from build123d import *

# Parameters (mm, degrees)
SKETCH1_W          = 16
SKETCH1_H          = 16
EXTRUDE1_DEPTH     = 8
SKETCH2_R          = 7.35
EXTRUDE2_DEPTH     = 7
SHELL1_T           = -1.3
SKETCH6_R          = 1
CUT_EXTRUDE1_DEPTH = 19.788294228
SKETCH4_R          = 1.15
EXTRUDE3_DEPTH     = 4
FILLET1_R          = 0.5
FILLET2_R          = 0.5
FILLET3_R          = 1


with BuildPart() as part:
    # Sketch1 → Extrude1 (new body)
    with BuildSketch(Plane.XY):
        Rectangle(SKETCH1_W, SKETCH1_H)
    extrude(amount=EXTRUDE1_DEPTH)

    # Sketch2 → Extrude2 (add)
    with BuildSketch(Plane.XY.offset(8)):
        Circle(SKETCH2_R)
    extrude(amount=EXTRUDE2_DEPTH)

    # Shell1
    shell1_openings = [part.faces().sort_by_distance(p)[0] for p in [
        (0, 0, 15),
        (0, 0, 0),
    ]]
    offset(amount=SHELL1_T, openings=shell1_openings, kind=Kind.INTERSECTION)

    # Sketch6 → Cut-Extrude1 (cut, through all)
    with BuildSketch(Plane(origin=(0, 0, 0), x_dir=(1, 0, 0), z_dir=(0, 1, 0))):
        with Locations(Location((0, -12.46, 0), (0, 0, 90))):
            Circle(SKETCH6_R)
    extrude(amount=CUT_EXTRUDE1_DEPTH, mode=Mode.SUBTRACT)

    # Sketch4 → Extrude3 (add)
    with BuildSketch(Plane.XY):
        with BuildLine():
            Line((-8, 1.9), (-10.3, 1.9))
            ThreePointArc((-10.3, 1.9), (-12.2, 0), (-10.3, -1.9))
            Line((-10.3, -1.9), (-8, -1.9))
            Line((-8, -1.9), (-8, 1.9))
        make_face()
        with Locations((-10.3, 0)):
            Circle(SKETCH4_R, mode=Mode.SUBTRACT)
        with BuildLine():
            Line((8, 1.9), (8, -1.9))
            Line((8, -1.9), (10.3, -1.9))
            ThreePointArc((10.3, -1.9), (12.2, 0), (10.3, 1.9))
            Line((10.3, 1.9), (8, 1.9))
        make_face()
        with Locations((10.3, 0)):
            Circle(SKETCH4_R, mode=Mode.SUBTRACT)
    extrude(amount=EXTRUDE3_DEPTH)

    # Fillet1
    fillet1_edges = [part.edges().sort_by_distance(p)[0] for p in [
        (-8, 8, 4),
        (-8, -8, 4),
        (8, -8, 4),
        (8, 8, 4),
        (0, -8, 8),
        (-8, 0, 8),
        (0, 8, 8),
        (8, 0, 8),
    ]]
    fillet(fillet1_edges, radius=FILLET1_R)

    # Fillet2
    fillet2_edges = [part.edges().sort_by_distance(p)[0] for p in [
        (-7.35, 0, 8),
        (-7.35, 0, 15),
    ]]
    fillet(fillet2_edges, radius=FILLET2_R)

    # Fillet3
    fillet3_edges = [part.edges().sort_by_distance(p)[0] for p in [
        (8, 1.9, 2),
        (8, -1.9, 2),
        (-8, -1.9, 2),
        (-8, 1.9, 2),
    ]]
    fillet(fillet3_edges, radius=FILLET3_R)


solid = part.part
Verification items for the finished model (mm, model axes). A direction names the side the tool comes from. Give positions to 0.01 mm unless a question says otherwise; leave off trailing zeros. Loops run counter-clockwise (first coordinate to the right, second up) from the corner with the lowest first, then second, coordinate; pieces in that order, holes last.
1. Cross-section at B-B on z = 12.46. Record the cut outline in (x, y), and give its area (3 significant figures).
Derived:
outline: (-1, 5.97) - (-1, 7.28) arc R7.35 ccw (long way) to (1, 7.28) - (1, 5.97) arc R6.05 cw (long way) to start
area: 52.1 mm2
2. Tool access check on faces 1 (the flat face through (10, 1.9, 2)), 2 (the cylindrical face through (11.397, 0.345, 1.972)), 3 (the flat face through (0, 6.7, 3)), 4 (the flat face through (9, 0, 4)), 5 (the flat face through (6, -6, 8)). Record the directions out of +Z, -Z, +X, -X, +Y, -Y that give a thin tool (end or side, any length) a straight path to the whole face; none if there is none.
Derived:
face 1: +Z, -Z, +X, +Y
face 2: +Z, -Z
face 3: -Z
face 4: +Z, +X, +Y, -Y
face 5: +Z, +X, -Y
3. Go/stop test with flat-tipped pins: P1, Ø1.3, axis at x = 10.5, y = -0.5, coming from the +Z side; P2, Ø1.4, axis at x = 9.5, z = 1.5, coming from the +Y side; P3, Ø2, axis at y = -2.5, z = 9.5, coming from the -X side. Record where each tip stops, or that it passes through.
Derived:
P1: stops at z = 4
P2: stops at y = 1.92
P3: stops at x = -7.2
4. Release check for a two-part mould opening along Y. For faces 6 (the flat face through (-6, 2, 6.7)), 7 (the cylindrical face through (7.01, 2.21, 11.41)), 8 (the flat face through (-8, 0, 5)), 9 (the cylindrical face through (-8.285, -2.201, 2.028)) record: +Y half, -Y half, draft (parallel to the pull), parting line (faces both ways), or undercut.
Derived:
face 6: undercut
face 7: parting line
face 8: draft
face 9: -Y half
5. Material ranges on probe 1 along Y at (x, z) = (-0.75, 3.5); probe 2 along Y at (x, z) = (-10.3, 2.1), recorded low to high.
Derived:
probe 1: y = -8 to -6.7, 6.7 to 8
probe 2: y = -1.9 to -1.15, 1.15 to 1.9
6. Cross-section at A-A on x = 0. Count the separate pieces of the cut face and the enclosed holes in it, and give its area (3 significant figures).
Derived:
separate pieces: 3
enclosed holes: 0
area: 37.9 mm2
7. Cross-section at C-C on x = -8.5. Record the cut outline in (y, z), and give its area (3 significant figures).
Derived:
outline: (-2.03, 0) - (2.03, 0) - (2.03, 4) - (-2.03, 4) - close
area: 16.3 mm2
